Input: dimensioned drawing with shaded views. Units: mm. Origin: part minimum x, y, z. Round coordinates to 2 decimals unless told otherwise and drop trailing zeros. Order: outer loops, then holes, each group sorted by start corner. A loop starts at its lowest first (then second) coordinate and runs counter-clockwise, first axis right, second up.
Item 1: Line query: L1, parallel to X at y = 1.35, z = 13.5; L2, parallel to X at y = 1.7, z = 22; L3, parallel to Z at x = 13, y = 2.4. Output: solid intervals per line, ascending.
Item 2: Cut plane B-B on x = 10. Output: boundary loops of the cut face in (y, z).
Item 3: Cut plane D-D on z = 22. Output: boundary loops of the cut face in (x, y), then the cut area to 3 significant figures.
Item 4: Cut plane A-A on z = 36. Output: boundary loops of the cut face in (x, y), then the cut area to 3 significant figures.
Item 5: Cut plane C-C on y = 2. Output: boundary loops of the cut face in (x, z).
Item 6: Mould query, pull axis Z, two halves, no side actions, for the marked faces 1 and 2. Classes: released by +Z, released by -Z, zero draft, split by the parting line, or undercut.
Item 7: First-contact query: pin 1 (1.5 mm diameter, centred on x = 10, z = 22, fed in from -Y). Flat tip, straight axial feed; report the tip coordinate or a pass-through.
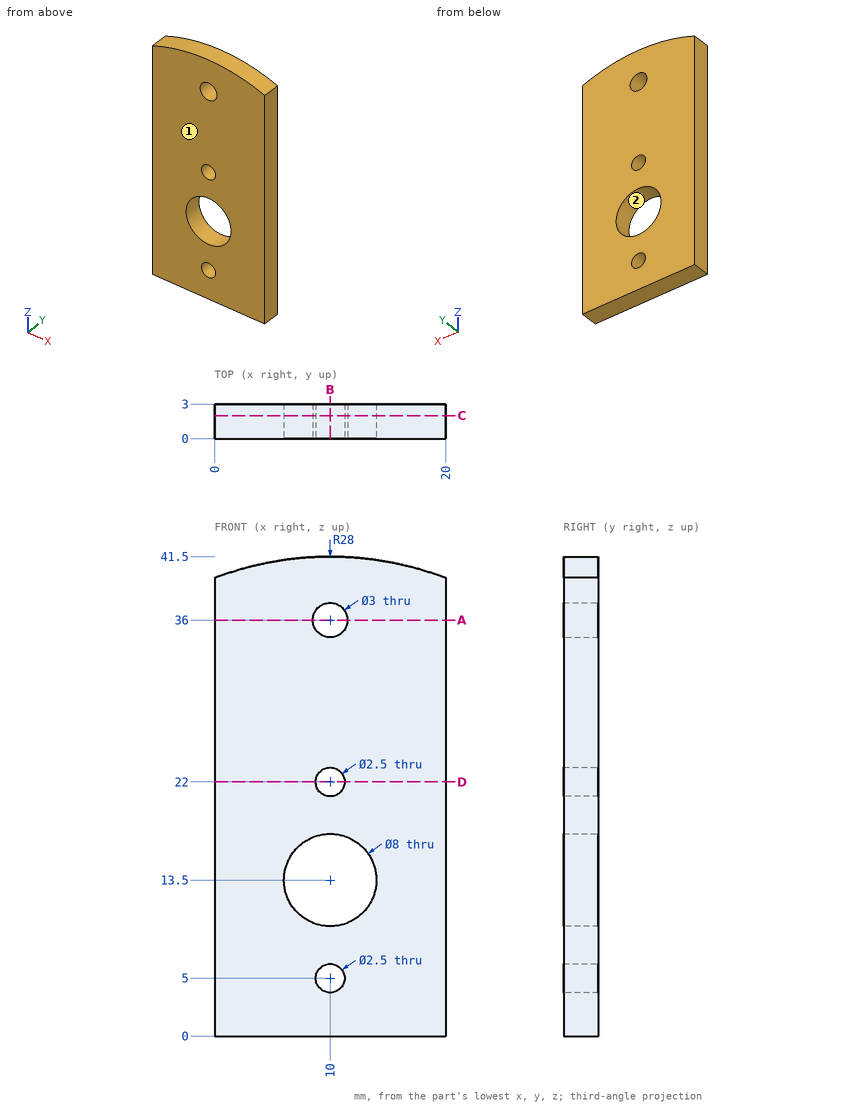
From the geometry:
1. L1: x = 0 to 6, 14 to 20
1. L2: x = 0 to 8.75, 11.25 to 20
1. L3: z = 0 to 10.85, 16.15 to 41.34
2. outline: (0, 0) - (3, 0) - (3, 3.75) - (0, 3.75) - close; (0, 6.25) - (3, 6.25) - (3, 9.5) - (0, 9.5) - close; (0, 17.5) - (3, 17.5) - (3, 20.75) - (0, 20.75) - close; (0, 23.25) - (3, 23.25) - (3, 34.5) - (0, 34.5) - close; (0, 37.5) - (3, 37.5) - (3, 41.5) - (0, 41.5) - close
3. outline: (0, 0) - (8.75, 0) - (8.75, 3) - (0, 3) - close; (11.25, 0) - (20, 0) - (20, 3) - (11.25, 3) - close
3. area: 52.5 mm2
4. outline: (0, 0) - (8.5, 0) - (8.5, 3) - (0, 3) - close; (11.5, 0) - (20, 0) - (20, 3) - (11.5, 3) - close
4. area: 51.0 mm2
5. outline: (0, 0) - (20, 0) - (20, 39.65) arc R28 ccw to (0, 39.65) - close; hole circle Ø8 at (10, 13.5); hole circle Ø3 at (10, 36); hole circle Ø2.5 at (10, 5); hole circle Ø2.5 at (10, 22)
6. face 1: zero draft
6. face 2: undercut
7. pin 1: passes through
